```python
from build123d import *

# Parameters (mm, degrees)
BOSS_EXTRU_6_DEPTH                 = 5
ESQUISSE4_R                        = 2
BOSS_EXTRU_5_DEPTH                 = 170
CONG_3_R                           = 2
R_P_TITION_CIRCULAIRE1_COUNT       = 2
R_P_TITION_CIRCULAIRE1_ANGLE       = 140
CONG_3_OF_R_P_TITION_CIRCULAIRE1_R = 2
ESQUISSE6_R                        = 2
ENL_V_MAT_EXTRU_2_DEPTH            = 202.524852693


with BuildPart() as part:
    # Esquisse1 → Boss.-Extru.6 (new body)
    with BuildSketch(Plane(origin=(0, 0, 0), x_dir=(1, 0, 0), z_dir=(0, 1, 0))):
        with BuildLine():
            ThreePointArc((0, -3), (3, 0), (0, 3))
            ThreePointArc((0, 3), (-3, 0), (0, -3))
        make_face()
    extrude(amount=BOSS_EXTRU_6_DEPTH)

    # Esquisse4 → Boss.-Extru.5 (add)
    with BuildSketch(Plane(origin=(0.427525179, 0.075384224, 0), x_dir=(0, 0, -1), z_dir=(0.984807753012208, 0.17364817766693072, 0))):
        with Locations(Location((0, 2, 0), (0, 0, 270))):
            Circle(ESQUISSE4_R)
    boss_extru_5 = extrude(amount=BOSS_EXTRU_5_DEPTH)

    # Congé3
    cong_3_edges = [part.edges().sort_by_distance(p)[0] for p in [
        (167.150250481, 33.534805439, 0),
    ]]
    fillet(cong_3_edges, radius=CONG_3_R)

    # Répétition circulaire1: Boss.-Extru.5 ×2 about axis
    r_p_tition_circulaire1_axis = Axis((0, 0, 0), (0, -1, 0))
    for i in range(1, R_P_TITION_CIRCULAIRE1_COUNT):
        add(boss_extru_5.rotate(r_p_tition_circulaire1_axis, i * R_P_TITION_CIRCULAIRE1_ANGLE / (R_P_TITION_CIRCULAIRE1_COUNT - 1)))

    # Congé3 of Répétition circulaire1
    cong_3_of_r_p_tition_circulaire1_edges = [part.edges().sort_by_distance(p)[0] for p in [
        (-128.044520547, 33.534805439, 107.442109965),
    ]]
    fillet(cong_3_of_r_p_tition_circulaire1_edges, radius=CONG_3_OF_R_P_TITION_CIRCULAIRE1_R)

    # Esquisse6 → Enlèv. mat.-Extru.2 (cut, through all)
    with BuildSketch(Plane(origin=(0, 5, 0), x_dir=(1, 0, 0), z_dir=(0, 1, 0))):
        with Locations(Location((0, 0, 0), (0, 0, 270))):
            Circle(ESQUISSE6_R)
    extrude(amount=-ENL_V_MAT_EXTRU_2_DEPTH, mode=Mode.SUBTRACT)


solid = part.part
```
The listing builds one solid part. Answer for the finished solid, in the listing's coordinates (mm). Give positions to 0.01 mm unless a question says otherwise; leave off trailing zeros.
1) Given P1, Ø1.5, axis at y = 24.5, z = 65, coming from the -X side; P2, Ø10, axis at x = -91.5, z = 82.5, coming from the -Y side; P3, Ø5, axis at x = 0, z = 1, coming from the +Y side; P4, Ø12, axis at x = 43, y = 16.5, coming from the -Z side, each flat-ended and moving along its own axis, determine where each tip first touches the part or whether it passes through.
Reported:
P1: passes through
P2: stops at y = 21.22
P3: stops at y = 5
P4: stops at z = -1.84
2) Consider line 1 along X through (y, z) = (10.5, 30.5); line 2 along Y through (x, z) = (-94.5, 79). Determine where each line is inside the solid, lowest interval first.
Reported:
line 1: x = -39.42 to -33.34
line 2: y = 21.73 to 25.77
3) Determine the mould class of faces 1 (the face through (-0.9, 2.46, -2.86)), 2 (the face through (2, 5, 1)), 3 (the face through (-63.046, 18.585, 53.016)) for opening direction X: pulls with the +X half, pulls with the -X half, needs draft (parallel to the pull), parting line crosses it, or undercut.
Reported:
face 1: undercut
face 2: needs draft
face 3: parting line crosses it
